Build history of the part. All positions in model axes, mm. A direction names the side the tool comes from. Round coordinates to 2 decimals unless told otherwise and drop trailing zeros. Write each loop counter-clockwise with the first axis right and the second up, starting at its lowest first coordinate (ties: lowest second). Pieces come first, ordered by that corner, then holes. Notation, with made-up numbers: (46.5, 72) -> (50.5, 72) arc R21 cw to (50.5, 76) -> close; hole circle Ø2 at (11, 54.5). An arc over 180 degrees is marked (long way). Return JSON: item names as keys, results as strings.
from build123d import *

# Parameters (mm, degrees)
F0_W     = 38.1
F0_H     = 107.95
F0_R     = 11.1125
F1_DEPTH = 3.175
F2_W     = 3.175
F2_H     = 6.35
F2_W_2   = 25.4
F2_H_2   = 44.45
F3_DEPTH = 3.175
F4_W     = 6.35
F4_H     = 3.175
F5_DEPTH = 3.175
F6_SIZE  = 4.7625


with BuildPart() as f1:
    # F0 (on Top) → F1 (new body)
    with BuildSketch(Plane.XY):
        with Locations((19.05, -53.975)):
            Rectangle(F0_W, F0_H)
        with Locations((19.05, -90.4875)):
            Circle(F0_R, mode=Mode.SUBTRACT)
        with Locations((19.05, -17.4625)):
            Circle(F0_R, mode=Mode.SUBTRACT)
    extrude(amount=F1_DEPTH)

    # F2 (on face) → F3 (cut, through all)
    with BuildSketch(Plane.XY.offset(3.175)):
        with Locations((36.5125, -3.175)):
            Rectangle(F2_W, F2_H)
        with Locations((1.5875, -3.175)):
            Rectangle(F2_W, F2_H)
        with Locations((1.5875, -15.875)):
            Rectangle(F2_W, F2_H)
        with Locations((36.5125, -15.875)):
            Rectangle(F2_W, F2_H)
        with Locations((36.5125, -28.575)):
            Rectangle(F2_W, F2_H)
        with Locations((36.5125, -41.275)):
            Rectangle(F2_W, F2_H)
        with Locations((36.5125, -53.975)):
            Rectangle(F2_W, F2_H)
        with Locations((36.5125, -66.675)):
            Rectangle(F2_W, F2_H)
        with Locations((36.5125, -79.375)):
            Rectangle(F2_W, F2_H)
        with Locations((36.5125, -92.075)):
            Rectangle(F2_W, F2_H)
        with Locations((36.5125, -104.775)):
            Rectangle(F2_W, F2_H)
        with Locations((36.5125, -117.475)):
            Rectangle(F2_W, F2_H)
        with Locations((36.5125, -130.175)):
            Rectangle(F2_W, F2_H)
        with Locations((1.5875, -28.575)):
            Rectangle(F2_W, F2_H)
        with Locations((1.5875, -41.275)):
            Rectangle(F2_W, F2_H)
        with Locations((1.5875, -53.975)):
            Rectangle(F2_W, F2_H)
        with Locations((1.5875, -66.675)):
            Rectangle(F2_W, F2_H)
        with Locations((1.5875, -79.375)):
            Rectangle(F2_W, F2_H)
        with Locations((1.5875, -92.075)):
            Rectangle(F2_W, F2_H)
        with Locations((1.5875, -104.775)):
            Rectangle(F2_W, F2_H)
        with Locations((1.5875, -117.475)):
            Rectangle(F2_W, F2_H)
        with Locations((1.5875, -130.175)):
            Rectangle(F2_W, F2_H)
        with Locations((19.05, -53.975)):
            Rectangle(F2_W_2, F2_H_2)
    extrude(amount=-F3_DEPTH, mode=Mode.SUBTRACT)

    # F4 (on face) → F5 (cut, through all)
    with BuildSketch(Plane.XY.offset(3.175)):
        with Locations((19.05, -1.5875)):
            Rectangle(F4_W, F4_H)
        with Locations((31.75, -1.5875)):
            Rectangle(F4_W, F4_H)
        with Locations((6.35, -1.5875)):
            Rectangle(F4_W, F4_H)
        with Locations((31.75, -106.3625)):
            Rectangle(F4_W, F4_H)
        with Locations((6.35, -106.3625)):
            Rectangle(F4_W, F4_H)
        with Locations((19.05, -106.3625)):
            Rectangle(F4_W, F4_H)
    extrude(amount=-F5_DEPTH, mode=Mode.SUBTRACT)

    # F6
    f6_edges = [f1.edges().sort_by_distance(p)[0] for p in [
        (31.75, -31.75, 1.5875),
        (6.35, -31.75, 1.5875),
        (6.35, -76.2, 1.5875),
        (31.75, -76.2, 1.5875),
    ]]
    chamfer(f6_edges, length=F6_SIZE)


solid = f1.part
Q1. Saw through at C-C on z = 1.55. Count the separate pieces of the cut face and the enclosed holes in it, then the cut area to 3 significant figures.
Verdict:
{"separate pieces": "1", "enclosed holes": "3", "area": "1,770 mm²"}
Q2. Pin check, flat tips, straight feed: pin 1 Ø1.5 at (x, z) = (6.5, 1) entering from -Y (3 decimals); pin 2 Ø1 at (x, z) = (1, 2) entering from -Y. Stop position of each tip, or through.
Verdict:
{"pin 1": "stops at y = -104.775", "pin 2": "stops at y = -101.6"}
Q3. Two-plate mould, pull along Y, no slides. Class faces 4 (the flat face through (2, -25.4, 2)), 5 (the flat face through (38.1, -98, 2)), 6 (the flat face through (36, -57.15, 2)), 7 (the flat face through (13, 0, 2)): +Y half, -Y half, draft (parallel to the pull), parting line (faces both ways), or undercut.
Verdict:
{"face 4": "undercut", "face 5": "draft", "face 6": "undercut", "face 7": "+Y half"}
Q4. Saw through at B-B on x = 4.5. List the corners of the cut face in (y, z) (3 decimals).
Verdict:
{"outline": "(-104.775, 0) -> (-3.175, 0) -> (-3.175, 3.175) -> (-104.775, 3.175) -> close"}
Q5. Saw through at A-A on x = 19.05. List the corners of the cut face in (y, z) (3 decimals).
Verdict:
{"outline": "(-104.775, 0) -> (-101.6, 0) -> (-101.6, 3.175) -> (-104.775, 3.175) -> close; (-79.375, 0) -> (-76.2, 0) -> (-76.2, 3.175) -> (-79.375, 3.175) -> close; (-31.75, 0) -> (-28.575, 0) -> (-28.575, 3.175) -> (-31.75, 3.175) -> close; (-6.35, 0) -> (-3.175, 0) -> (-3.175, 3.175) -> (-6.35, 3.175) -> close"}
Q6. Wall check: L1, parallel to Y at x = 19.05, z = 1 (3 decimals); L2, parallel to Y at x = 9, z = 0.65 (1 decimal); L3, parallel to X at y = -43, z = 1.6 (3 decimals). Give the ranges that are in metal, low to high.
Verdict:
{"L1": "y = -104.775 to -101.6, -79.375 to -76.2, -31.75 to -28.575, -6.35 to -3.175", "L2": "y = -104.8 to -95.2, -85.7 to -74.1, -33.9 to -22.2, -12.7 to -3.2", "L3": "x = 3.175 to 6.35, 31.75 to 34.925"}
Q7. 3-axis set-ups, long thin cutter, end or side, ignore diameter. For faces 1 (the flat face through (28.575, -2, 2)), 2 (the flat face through (3.175, -16, 2)), 3 (the flat face through (2, -6.35, 2)): which of +Z, -Z, +X, -X, +Y, -Y reach the whole face in a straight line?
Verdict:
{"face 1": "+Z, -Z, +X, +Y", "face 2": "+Z, -Z, -X", "face 3": "+Z, -Z, -X, +Y"}
